Verification items for the finished model (mm, model axes). Round coordinates to 2 decimals unless told otherwise and drop trailing zeros. Write each loop counter-clockwise with the first axis right and the second up, starting at its lowest first coordinate (ties: lowest second). Pieces come first, ordered by that corner, then holes. Notation, with made-up numbers: (-31.75, 7.5) - (1.25, 7.5) arc R32 ccw to (1.25, 33.5) - close; hole circle Ø1 at (-15, 8.25). An arc over 180 degrees is marked (long way). Answer as a JSON object with one key per item and string values.
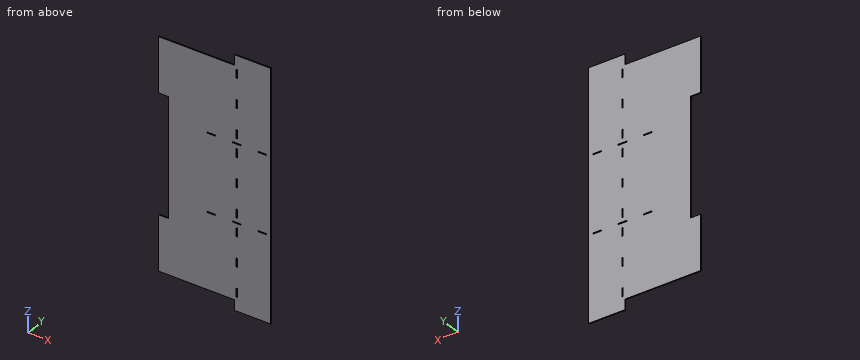
```python
from build123d import *

# Parameters (mm, degrees)
SKETCH3_W           = 25.4
SKETCH3_H           = 3.175
SKETCH3_W_2         = 3.175
SKETCH3_H_2         = 25.4
BOSS_EXTRUDE1_DEPTH = 3.175
SKETCH6_W           = 107.287119944
SKETCH6_H           = 30.1625
SKETCH6_W_2         = 30.1625
SKETCH6_H_2         = 160.930679916
BOSS_EXTRUDE2_DEPTH = 3.175


with BuildPart() as part:
    # Sketch3 → Boss-Extrude1 (new body)
    with BuildSketch(Plane(origin=(0, 0, 0), x_dir=(1, 0, 0), z_dir=(0, 1, 0))):
        Polygon((0, 0), (200.98004, 0), (200.98004, 669.93516), (0, 669.93516), (-100.8126, 669.93516), (-100.8126, 0), align=None)
        with Locations((25.4, 448.21094)):
            Rectangle(SKETCH3_W, SKETCH3_H, mode=Mode.SUBTRACT)
        with Locations((175.58004, 448.21094)):
            Rectangle(SKETCH3_W, SKETCH3_H, mode=Mode.SUBTRACT)
        with Locations((100.49002, 448.21094)):
            Rectangle(SKETCH3_W, SKETCH3_H, mode=Mode.SUBTRACT)
        with Locations((100.49002, 647.71016)):
            Rectangle(SKETCH3_W_2, SKETCH3_H_2, mode=Mode.SUBTRACT)
        with Locations((100.49002, 475.19844)):
            Rectangle(SKETCH3_W_2, SKETCH3_H_2, mode=Mode.SUBTRACT)
        with Locations((100.49002, 561.4543)):
            Rectangle(SKETCH3_W_2, SKETCH3_H_2, mode=Mode.SUBTRACT)
        with Locations((100.49002, 421.22344)):
            Rectangle(SKETCH3_W_2, SKETCH3_H_2, mode=Mode.SUBTRACT)
        with Locations((100.49002, 334.96758)):
            Rectangle(SKETCH3_W_2, SKETCH3_H_2, mode=Mode.SUBTRACT)
        with Locations((100.49002, 248.71172)):
            Rectangle(SKETCH3_W_2, SKETCH3_H_2, mode=Mode.SUBTRACT)
        with Locations((25.4, 221.72422)):
            Rectangle(SKETCH3_W, SKETCH3_H, mode=Mode.SUBTRACT)
        with Locations((100.49002, 221.72422)):
            Rectangle(SKETCH3_W, SKETCH3_H, mode=Mode.SUBTRACT)
        with Locations((175.58004, 221.72422)):
            Rectangle(SKETCH3_W, SKETCH3_H, mode=Mode.SUBTRACT)
        with Locations((100.49002, 22.225)):
            Rectangle(SKETCH3_W_2, SKETCH3_H_2, mode=Mode.SUBTRACT)
        with Locations((100.49002, 108.48086)):
            Rectangle(SKETCH3_W_2, SKETCH3_H_2, mode=Mode.SUBTRACT)
        with Locations((100.49002, 194.73672)):
            Rectangle(SKETCH3_W_2, SKETCH3_H_2, mode=Mode.SUBTRACT)
    extrude(amount=BOSS_EXTRUDE1_DEPTH)

    # Sketch6 → Boss-Extrude2 (add)
    with BuildSketch(Plane(origin=(0, 3.175, 0), x_dir=(1, 0, 0), z_dir=(0, 1, 0))):
        with Locations((147.336480028, -15.08125)):
            Rectangle(SKETCH6_W, SKETCH6_H)
        with Locations((147.336480028, 685.01641)):
            Rectangle(SKETCH6_W, SKETCH6_H)
        with Locations((-115.89385, 589.469820042)):
            Rectangle(SKETCH6_W_2, SKETCH6_H_2)
        with Locations((-115.89385, 80.465339958)):
            Rectangle(SKETCH6_W_2, SKETCH6_H_2)
    extrude(amount=-BOSS_EXTRUDE2_DEPTH)


solid = part.part
```
1. Cross-section at A-A (y = 1.6). Count the separate pieces of the cut face and the enclosed holes in it, plus the area to 3 significant figures.
Completed:
{"separate pieces": "1", "enclosed holes": "15", "area": "217,000 mm^2"}
2. Cross-section at C-C (x = 1). Record the boundary of the cut face in (y, z) (3 decimals), plus the area to 3 significant figures.
Completed:
{"outline": "(0, -669.935) - (3.175, -669.935) - (3.175, 0) - (0, 0) - close", "area": "2,130 mm^2"}
3. Cross-section at B-B (z = -307). Record the boundary of the cut face in (x, y) (3 decimals), plus the area to 3 significant figures.
Completed:
{"outline": "(-100.813, 0) - (200.98, 0) - (200.98, 3.175) - (-100.813, 3.175) - close", "area": "958 mm^2"}
4. Material ranges on probe 1 along Z at (x, y) = (103, 1.65); probe 2 along Z at (x, y) = (32, 1.85); probe 3 along X at (y, z) = (2.85, -646), recorded low to high. Write a range as from..to.
Completed:
{"probe 1": "z = -700.1..-449.8, -446.62..-223.31, -220.14..30.16", "probe 2": "z = -669.94..-449.8, -446.62..-223.31, -220.14..0", "probe 3": "x = -130.98..98.9, 102.08..200.98"}
5. Go/stop test with flat-tipped pins: pin 1 (12 mm diameter, centred on x = 109, z = -622.5, fed in from -Y); pin 2 (1 mm diameter, centred on y = 1, z = -447.5, fed in from -X). Record where each tip stops, or that it passes through.
Completed:
{"pin 1": "stops at y = 0", "pin 2": "stops at x = -100.81"}
